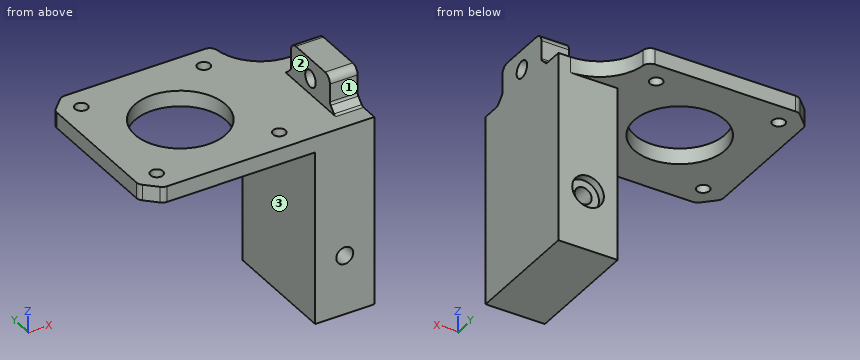
from build123d import *

# Parameters (mm, degrees)
CROQUIS1_R              = 1.6
CROQUIS1_R_2            = 11.5
SALIENTE_EXTRUIR1_DEPTH = 4
CROQUIS2_W              = 9
CROQUIS2_H              = 16
CROQUIS2_R              = 2.15
SALIENTE_EXTRUIR2_DEPTH = 7
CROQUIS3_W              = 15
CROQUIS3_H              = 42.2
SALIENTE_EXTRUIR3_DEPTH = 44
CORTAR_EXTRUIR1_START   = -12.3
CROQUIS4_W              = 15
CROQUIS4_H              = 48
CORTAR_EXTRUIR1_DEPTH   = 12.3
REDONDEO1_R             = 12
REDONDEO2_R             = 2
REDONDEO3_R             = 2
CHAFL_N1_SIZE           = 2
CHAFL_N2_SIZE           = 2
REDONDEO4_R             = 2
REDONDEO5_R             = 1
CROQUIS5_R              = 2.15
CORTAR_EXTRUIR2_DEPTH   = 30.9000001
CROQUIS5_3_R            = 4
CROQUIS5_3_R_2          = 2.15
CORTAR_EXTRUIR3_DEPTH   = 2


with BuildPart() as part:
    # Croquis1 → Saliente-Extruir1 (new body)
    with BuildSketch(Plane.XY):
        Polygon((21.15, 21.15), (17.15, 21.15), (-17.15, 21.15), (-21.15, 17.15), (-21.15, -17.15), (-17.15, -21.05), (17.15, -21.05), (36.15, -21.05), (36.15, 21.15), align=None)
        with Locations((-15.5, 15.5)):
            Circle(CROQUIS1_R, mode=Mode.SUBTRACT)
        with Locations((-15.5, -15.5)):
            Circle(CROQUIS1_R, mode=Mode.SUBTRACT)
        with Locations((15.5, 15.5)):
            Circle(CROQUIS1_R, mode=Mode.SUBTRACT)
        with Locations((15.5, -15.5)):
            Circle(CROQUIS1_R, mode=Mode.SUBTRACT)
        Circle(CROQUIS1_R_2, mode=Mode.SUBTRACT)
    extrude(amount=SALIENTE_EXTRUIR1_DEPTH)

    # Croquis2 → Saliente-Extruir2 (add)
    with BuildSketch(Plane(origin=(36.15, 0, 0), x_dir=(0, 0, -1), z_dir=(1, 0, 0))):
        with Locations((-8.5, -6.15)):
            Rectangle(CROQUIS2_W, CROQUIS2_H)
        with Locations((-8, -6.15)):
            Circle(CROQUIS2_R, mode=Mode.SUBTRACT)
    extrude(amount=-SALIENTE_EXTRUIR2_DEPTH)

    # Croquis3 → Saliente-Extruir3 (add)
    with BuildSketch(Plane(origin=(0, 0, 0), x_dir=(-1, 0, 0), z_dir=(0, 0, -1))):
        with Locations((-28.65, 0.05)):
            Rectangle(CROQUIS3_W, CROQUIS3_H)
    extrude(amount=SALIENTE_EXTRUIR3_DEPTH)

    # Croquis4 → Cortar-Extruir1 (cut)
    with BuildSketch(Plane(origin=(0, 21.15, 0), x_dir=(1, 0, 0), z_dir=(0, 1, 0)).offset(CORTAR_EXTRUIR1_START)):
        with Locations((28.65, 20)):
            Rectangle(CROQUIS4_W, CROQUIS4_H)
    extrude(amount=CORTAR_EXTRUIR1_DEPTH, mode=Mode.SUBTRACT)

    # Redondeo1
    redondeo1_edges = [part.edges().sort_by_distance(p)[0] for p in [
        (21.15, 8.85, 2),
    ]]
    fillet(redondeo1_edges, radius=REDONDEO1_R)

    # Redondeo2
    redondeo2_edges = [part.edges().sort_by_distance(p)[0] for p in [
        (21.15, 21.15, 2),
    ]]
    fillet(redondeo2_edges, radius=REDONDEO2_R)

    # Redondeo3
    redondeo3_edges = [part.edges().sort_by_distance(p)[0] for p in [
        (-17.15, -21.05, 2),
        (-21.15, -17.15, 2),
        (-21.15, 17.15, 2),
        (-17.15, 21.15, 2),
    ]]
    fillet(redondeo3_edges, radius=REDONDEO3_R)

    # Chaflán1
    chafl_n1_edges = [part.edges().sort_by_distance(p)[0] for p in [
        (32.65, 1.85, 4),
    ]]
    chamfer(chafl_n1_edges, length=CHAFL_N1_SIZE)

    # Chaflán2
    chafl_n2_edges = [part.edges().sort_by_distance(p)[0] for p in [
        (32.65, -14.15, 4),
    ]]
    chamfer(chafl_n2_edges, length=CHAFL_N2_SIZE)

    # Redondeo4
    redondeo4_edges = [part.edges().sort_by_distance(p)[0] for p in [
        (32.65, 1.85, 13),
        (32.65, -14.15, 13),
    ]]
    fillet(redondeo4_edges, radius=REDONDEO4_R)

    # Redondeo5
    redondeo5_edges = [part.edges().sort_by_distance(p)[0] for p in [
        (32.65, 3.85, 4),
        (32.65, 1.85, 6),
        (32.65, -14.15, 6),
        (32.65, -16.15, 4),
    ]]
    fillet(redondeo5_edges, radius=REDONDEO5_R)

    # Croquis5 → Cortar-Extruir2 (cut, through all)
    with BuildSketch(Plane(origin=(0, 8.85, 0), x_dir=(1, 0, 0), z_dir=(0, 1, 0))):
        with Locations((28.65, 29)):
            Circle(CROQUIS5_R)
    extrude(amount=-CORTAR_EXTRUIR2_DEPTH, mode=Mode.SUBTRACT)

    # Croquis5<3> → Cortar-Extruir3 (cut)
    with BuildSketch(Plane(origin=(0, 8.85, 0), x_dir=(1, 0, 0), z_dir=(0, 1, 0))):
        with Locations((28.65, 29)):
            Circle(CROQUIS5_3_R)
        with Locations((28.65, 29)):
            Circle(CROQUIS5_3_R_2, mode=Mode.SUBTRACT)
    extrude(amount=-CORTAR_EXTRUIR3_DEPTH, mode=Mode.SUBTRACT)


solid = part.part
The model under review builds one solid part; all positions refer to its coordinate system, in mm. Face numbers are marked on the shaded views. A direction names the side the tool comes from. Round coordinates to 2 decimals unless told otherwise and drop trailing zeros. Loops run counter-clockwise (first coordinate to the right, second up) from the corner with the lowest first, then second, coordinate; pieces in that order, holes last. Notation, with made-up numbers: (89.25, 32.5) -> (108.25, 32.5) arc R20 ccw to (108.25, 45.5) -> close; hole circle Ø3 at (-28, -12). An arc over 180 degrees is marked (long way). One line per question, with ' | ' between items. Start each with the question number.
Item 1: Add section A-A, the plane z = -29. Write out the cut boundary in (x, y).
Item 2: Wall thickness on line 1 along Y through (x, z) = (-15.5, 2.7); line 2 along X through (y, z) = (-10.25, -29); line 3 along Z through (x, y) = (32, -6): over which ranges is each line inside the solid? List them lowest first. Write a range as [from, to].
Item 3: Add section B-B, the plane x = 15.5. Write out the cut boundary in (y, z).
Item 4: For pin 1 (5 mm diameter, centred on x = 34, z = 8, fed in from -Y); pin 2 (12 mm diameter, centred on x = -11.5, y = 14.5, fed in from -Z); pin 3 (2.5 mm diameter, centred on y = -10, z = 9, fed in from -X); pin 4 (2.5 mm diameter, centred on x = 15.5, y = 15.5, fed in from +Z), all flat-tipped, find the tip position at first contact; note any pin that passes through.
Item 5: Machinability: for the marked faces 1, 2 and 3, which of the approach directions +Z, -Z, +X, -X, +Y, -Y give a long, thin tool a straight path to every point of the face, cutting with its end or side? Answer none if there is none.
Item 6: Add section D-D, the plane x = -2. Write out the cut boundary in (y, z).
Item 7: Add section C-C, the plane y = -2.5. Write out the cut boundary in (x, z).
Return value:
1) outline: (21.15, -21.05) -> (26.5, -21.05) -> (26.5, 6.85) -> (24.65, 6.85) -> (24.65, 8.85) -> (21.15, 8.85) -> close; (30.8, -21.05) -> (36.15, -21.05) -> (36.15, 8.85) -> (32.65, 8.85) -> (32.65, 6.85) -> (30.8, 6.85) -> close
2) line 1: y = [-21.05, -17.1], [-13.9, 13.9], [17.1, 21.15] | line 2: x = [21.15, 26.5], [30.8, 36.15] | line 3: z = [-44, 5.86], [10.14, 13]
3) outline: (-21.05, 0) -> (-17.1, 0) -> (-17.1, 4) -> (-21.05, 4) -> close; (-13.9, 0) -> (13.9, 0) -> (13.9, 4) -> (-13.9, 4) -> close; (17.1, 0) -> (21.15, 0) -> (21.15, 4) -> (17.1, 4) -> close
4) pin 1: stops at y = -14.65 | pin 2: stops at z = 0 | pin 3: stops at x = 29.15 | pin 4: passes through
5) face 1: +Z, +X, -X, -Y | face 2: +Z, -X, +Y, -Y | face 3: -Z, -X, +Y, -Y
6) outline: (-21.05, 0) -> (-11.32, 0) -> (-11.32, 4) -> (-21.05, 4) -> close; (11.32, 0) -> (21.15, 0) -> (21.15, 4) -> (11.32, 4) -> close
7) outline: (-21.15, 0) -> (-11.22, 0) -> (-11.22, 4) -> (-21.15, 4) -> close; (11.22, 0) -> (21.15, 0) -> (21.15, -44) -> (36.15, -44) -> (36.15, 13) -> (29.15, 13) -> (29.15, 4) -> (11.22, 4) -> close; hole circle Ø4.3 at (28.65, -29)
